```python
from build123d import *

# Parameters (mm, degrees)
SKETCH1_R           = 4.2
BOSS_EXTRUDE1_DEPTH = 10


with BuildPart() as part:
    # Sketch1 → Boss-Extrude1 (new body)
    with BuildSketch(Plane(origin=(0, 0, 0), x_dir=(1, 0, 0), z_dir=(0, 1, 0))):
        Polygon((0, 9.814954576), (-8.5, 4.907477288), (-8.5, -4.907477288), (0, -9.814954576), (8.5, -4.907477288), (8.5, 4.907477288), align=None)
        Circle(SKETCH1_R, mode=Mode.SUBTRACT)
    extrude(amount=BOSS_EXTRUDE1_DEPTH)

    # Sketch2 → Cut-Revolve1 (revolve, cut)
    with BuildSketch(Plane(origin=(0, 0, 0), x_dir=(0, 0, -1), z_dir=(1, 0, 0))):
        Polygon((-9.814954576, 9), (-7.361215932, 10), (-9.814954576, 10), align=None)
        Polygon((-7.361215932, 0), (-9.814954576, 0), (-9.814954576, 1), align=None)
    revolve(axis=Axis((0, 13.206770677, 0), (0, -1, 0)), mode=Mode.SUBTRACT)


solid = part.part
```
The model under review builds one solid part; all positions refer to its coordinate system, in mm. Give positions to 0.01 mm unless a question says otherwise; leave off trailing zeros. Write each loop counter-clockwise with the first axis right and the second up, starting at its lowest first coordinate (ties: lowest second). Pieces come first, ordered by that corner, then holes. Notation, with made-up numbers: M 33.25,20 L 88.25,20 A18 ccw 88.25,41 Z; hole C 46.25,24.25 d1. An arc over 180 degrees is marked long. Write each question's results on one line, items separated by ' | '. Start each with the question number.
1. We need section A-A (z = 0). Write out the cut boundary in (x, y).
2. Mouldability with a two-part tool opening along Z and no side actions: class faces 1 (the flat face through (3.2, 10, 3.2)), 2 (the cylindrical face through (4.006, 4.93, -1.262)), 3 (the flat face through (-4.191, 4.936, -7.396)) as released by +Z, released by -Z, zero draft, split by the parting line, or undercut.
3. For probe 1 along X at (y, z) = (5.25, 0); probe 2 along X at (y, z) = (6.5, 1.75); probe 3 along Z at (x, y) = (-3.75, 5), list the stretches that pass through material, from the lowest coordinate up. Write a range as [from, to].
4. We need section B-B (y = 4.75). Write out the cut boundary in (x, z), and give its area (3 significant figures).
5. Insertion check: pin 1 Ø6.5 at (x, z) = (0, 0) entering from -Y; pin 2 Ø5 at (x, y) = (6, 5.5) entering from -Z. Each pin has a flat end and moves straight along its axis. Give the tip position at first contact, or say it passes through.
Results found:
1) outline: M -8.5,0.46 L -7.36,0 L -4.2,0 L -4.2,10 L -7.36,10 L -8.5,9.54 Z; M 4.2,0 L 7.36,0 L 8.5,0.46 L 8.5,9.54 L 7.36,10 L 4.2,10 Z
2) face 1: zero draft | face 2: undercut | face 3: released by -Z
3) probe 1: x = [-8.5, -4.2], [4.2, 8.5] | probe 2: x = [-8.5, -3.82], [3.82, 8.5] | probe 3: z = [-7.65, -1.89], [1.89, 7.65]
4) outline: M -8.5,-4.91 L 0,-9.81 L 8.5,-4.91 L 8.5,4.91 L 0,9.81 L -8.5,4.91 Z; hole C 0,0 d8.4 | area: 195 mm^2
5) pin 1: passes through | pin 2: stops at z = -7.79
